The drawing under review shows one solid part. Ordinate dimensions are in mm from its lowest x, y, z. A direction names the side the tool comes from. Coordinates: 2 decimals unless noted, no trailing zeros. Write each loop counter-clockwise with the first axis right and the second up, starting at its lowest first coordinate (ties: lowest second). Pieces come first, ordered by that corner, then holes.
1) Add section B-B, the plane y = 170. State the section outline as (x, z) points.
2) Add section C-C, the plane x = 45. State the section outline as (y, z) points, then the cut area to 3 significant figures.
3) Add section A-A, the plane z = 184.5. State the section outline as (x, y) points.
4) For line 1 (X direction, y = 187.5, z = 275); line 2 (Y direction, x = 15, z = 312); line 3 (Y direction, x = 179, z = 253) (3 decimals), list the stretches that pass through material, from the lowest coordinate up.
5) Add section D-D, the plane z = 250. State the section outline as (x, y) points.
6) Mouldability with a two-part tool opening along X and no side actions: class the marked faces 4, 5 and 6 as released by +X, released by -X, zero draft, split by the parting line, or undercut.
7) Machinability: for the marked faces 1, 2 and 3, which of the approach directions +Z, -Z, +X, -X, +Y, -Y give a long, thin tool a straight path to every point of the face, cutting with its end or side? Answer none if there is none.
8) For P1, Ø10, axis at y = 322, z = 137.5, coming from the +X side; P2, Ø6, axis at x = 24.5, y = 167, coming from the +Z side; P3, Ø5, axis at x = 166.5, z = 158.5, coming from the -Y side, all flat-tipped, find the tip position at first contact; note any pin that passes through.
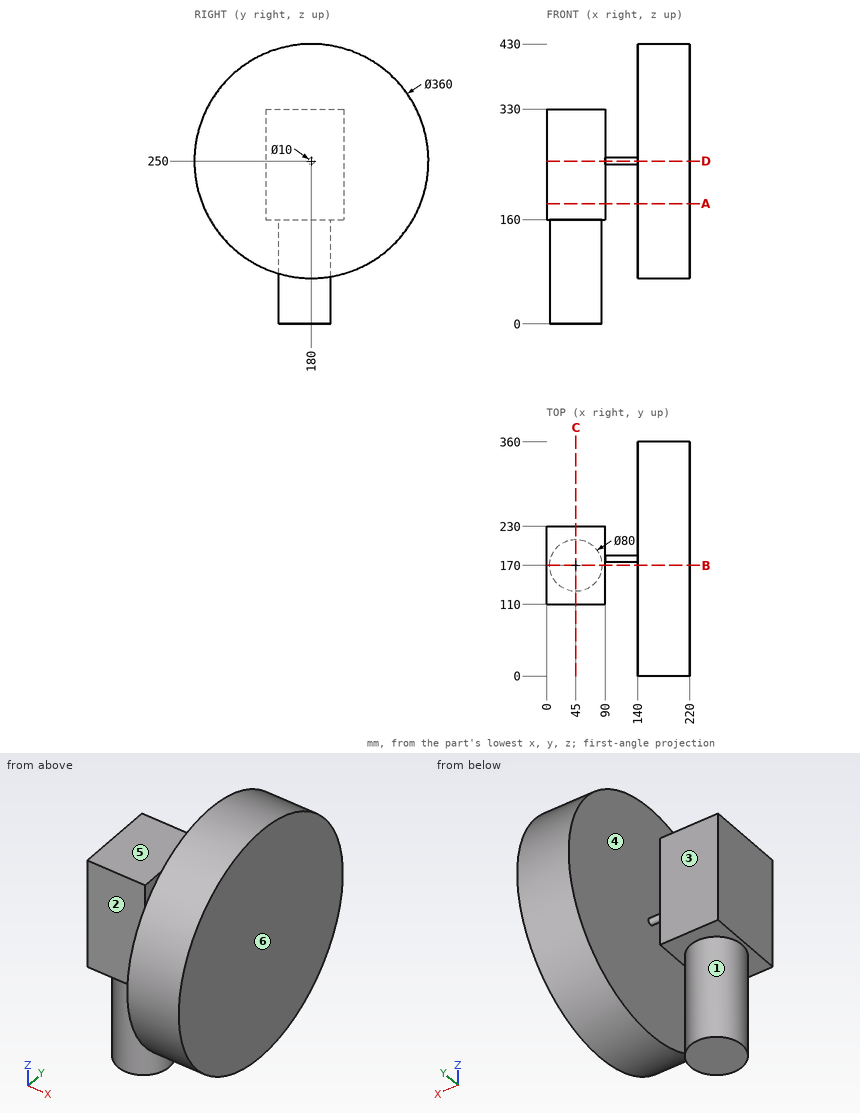
Geometry results:
1. outline: (0, 160) - (5, 160) - (5, 0) - (85, 0) - (85, 160) - (90, 160) - (90, 330) - (0, 330) - close; (140, 70.28) - (220, 70.28) - (220, 429.72) - (140, 429.72) - close
2. outline: (110, 160) - (130, 160) - (130, 0) - (210, 0) - (210, 160) - (230, 160) - (230, 330) - (110, 330) - close
2. area: 33,200 mm2
3. outline: (0, 110) - (90, 110) - (90, 230) - (0, 230) - close; (140, 12.34) - (220, 12.34) - (220, 347.66) - (140, 347.66) - close
4. line 1: x = 0 to 90, 140 to 220
4. line 2: y = 110 to 230
4. line 3: y = 0.025 to 359.975
5. outline: (0, 110) - (90, 110) - (90, 175) - (140, 175) - (140, 0) - (220, 0) - (220, 360) - (140, 360) - (140, 185) - (90, 185) - (90, 230) - (0, 230) - close
6. face 4: undercut
6. face 5: zero draft
6. face 6: released by +X
7. face 1: -Z
7. face 2: +Z, -Z, -X, -Y
7. face 3: +Z, -Z, -X, +Y
8. P1: stops at x = 220
8. P2: stops at z = 330
8. P3: stops at y = 23.54
